```python
from build123d import *

# Parameters (mm, degrees)
F0_R          = 5.4
F0_R_2        = 5
F1_DEPTH      = 62
F1_DEPTH_BACK = 9
F5_R          = 5
F6_DEPTH      = 1
F7_R          = 1
F8_R          = 0.2
F9_R          = 0.2


# Not quite as in the source:
# - a feature names something its author has since deleted; it is built from what else it names


with BuildPart() as f1:
    # F0 (on Top) → F1 (new body, two sides)
    with BuildSketch(Plane.XY) as f1_sk:
        Circle(F0_R)
        Circle(F0_R_2, mode=Mode.SUBTRACT)
    extrude(amount=F1_DEPTH)
    extrude(f1_sk.sketch, amount=-F1_DEPTH_BACK)

    # F2 (on Front) → F3 (revolve)
    with BuildSketch(Plane.XZ):
        with BuildLine():
            Line((6, 62), (4.6430466171, 62.5427813535))
            ThreePointArc((4.6430466171, 62.5427813535), (2.3596638473, 64.3820207615), (1.5, 67.1851648075))
            Line((1.5, 67.1851648075), (1.5, 72))
            Line((1.5, 72), (0.5, 72))
            Line((0.5, 72), (0.5, 63.8000000012))
            Line((0.5, 63.8000000012), (5, 62))
            Line((5, 62), (6, 62))
        make_face()
    revolve(axis=Axis((0, 0, 62.4439572394), (0, 0, 1)))

    # F5 (on offset) → F6 (join)
    with BuildSketch(Plane(origin=(0, 0, -9), x_dir=(1, 0, 0), z_dir=(0, 0, -1))):
        Polygon((11, 3.3135847191), (4.4980677776, 5.7), (-4.4980677776, 5.7), (-11, 3.3135847191), (-11, -2.1135847191), (-4.4980677776, -5.7), (4.4980677776, -5.7), (11, -2.1135847191), align=None)
        Circle(F5_R, mode=Mode.SUBTRACT)
    extrude(amount=F6_DEPTH)

    # F7
    f7_edges = [f1.edges().sort_by_distance(p)[0] for p in [
        (11, 2.113585, -9.5),
        (11, -3.313585, -9.5),
        (4.498068, 5.7, -9.5),
        (4.498068, -5.7, -9.5),
        (-4.498068, 5.7, -9.5),
        (-4.498068, -5.7, -9.5),
        (-11, 2.113585, -9.5),
        (-11, -3.313585, -9.5),
    ]]
    fillet(f7_edges, radius=F7_R)

    # F8
    f8_edges = [f1.edges().sort_by_distance(p)[0] for p in [
        (-7.504731, -4.596459, -10),
        (-4.495326, -5.684572, -10),
        (0, -5.7, -10),
        (-11, -0.546125, -10),
        (-10.819926, -3.187857, -10),
        (-10.861101, 2.031572, -10),
        (-7.603269, 3.987195, -10),
        (-4.489932, 5.668408, -10),
        (0, 5.7, -10),
        (4.489932, 5.668408, -10),
        (7.603269, 3.987195, -10),
        (7.504731, -4.596459, -10),
        (4.495326, -5.684572, -10),
        (10.819926, -3.187857, -10),
        (11, -0.546125, -10),
        (10.861101, 2.031572, -10),
    ]]
    fillet(f8_edges, radius=F8_R)

    # F9
    f9_edges = [f1.edges().sort_by_distance(p)[0] for p in [
        (10.819926, -3.187857, -9),
        (11, -0.546125, -9),
        (10.861101, 2.031572, -9),
        (7.603269, 3.987195, -9),
        (4.489932, 5.668408, -9),
        (0, 5.7, -9),
        (-4.489932, 5.668408, -9),
        (-10.861101, 2.031572, -9),
        (-7.603269, 3.987195, -9),
        (7.504731, -4.596459, -9),
        (0, -5.7, -9),
        (-11, -0.546125, -9),
        (-10.819926, -3.187857, -9),
        (-4.495326, -5.684572, -9),
        (4.495326, -5.684572, -9),
        (-7.504731, -4.596459, -9),
    ]]
    fillet(f9_edges, radius=F9_R)


solid = f1.part
```
The model under review builds one solid part; all positions refer to its coordinate system, in mm. A direction names the side the tool comes from. Round coordinates to 2 decimals unless told otherwise and drop trailing zeros. Order: outer loops, then holes, each group sorted by start corner. A loop starts at its lowest first (then second) coordinate and runs counter-clockwise, first axis right, second up. Notation, with made-up numbers: M 43,-3.75 L 62,-3.75 A22 cw 62,19.25 Z; hole C 34,74 d9. An arc over 180 degrees is marked long. Use a Markdown table: item, result.
1) Tool access review of faces 1 (the face through (-1.5, 0.07, 69.63)), 2 (the face through (7.615, 3.912, -9.943)): name each direction out of +Z, -Z, +X, -X, +Y, -Y from which nothing blocks a thin tool from reaching the whole face with its end or side.
Report:
| item | result |
|---|---|
| face 1 | +Z |
| face 2 | -Z, +X, +Y |
2) Insertion check: pin 1 (2 mm diameter, centred on x = -1, y = -3.5, fed in from -Z); pin 2 (0.5 mm diameter, centred on x = -0.5, z = -9.5, fed in from -Y); pin 3 (5 mm diameter, centred on y = 4, z = -0.5, fed in from -X). Each pin has a flat end and moves straight along its axis. Give the tip position at first contact, or say it passes through.
Report:
| item | result |
|---|---|
| pin 1 | z = 62.14 |
| pin 2 | y = -5.7 |
| pin 3 | x = -5.19 |
3) Wall thickness on line 1 along Y through (x, z) = (0, -6); line 2 along X through (y, z) = (2, 43); line 3 along Y through (x, z) = (0, -9.3): over which ranges is each line inside the solid? List them lowest first. Write a range as [from, to].
Report:
| item | result |
|---|---|
| line 1 | [-5.4, -5], [5, 5.4] |
| line 2 | [-5.02, -4.58], [4.58, 5.02] |
| line 3 | [-5.7, -5], [5, 5.7] |
4) Consider section A-A (z = 59). Write out the cut boundary in (x, y), then the cut area to 3 significant figures.
Report:
| item | result |
|---|---|
| outline | C 0,0 d10.8; hole C 0,0 d10 |
| area | 13.1 mm^2 |
5) Draft analysis for pull direction Z (two halves, no side actions). For faces 3 (the face through (-7.53, 3.96, -9.94)), 4 (the face through (-1.17, -5.27, 27)), 5 (the face through (-7.616, 3.915, -9.06)), state which applies: released by +Z, released by -Z, zero draft, split by the parting line, or undercut.
Report:
| item | result |
|---|---|
| face 3 | released by -Z |
| face 4 | undercut |
| face 5 | released by +Z |
